Input: part model. Units: mm. Frame: model coordinates. Face numbers are marked on the shaded views. A direction names the side the tool comes from. Give positions to 0.01 mm unless a question says otherwise; leave off trailing zeros. Loops run counter-clockwise (first coordinate to the right, second up) from the corner with the lowest first, then second, coordinate; pieces in that order, holes last. Notation, with made-up numbers: (35, -16) -> (82, -16) arc R15 cw to (82, 5) -> close; hole circle Ø10 at (-22.75, 68.5). An arc over 180 degrees is marked (long way). One line per question, with ' | ' between items.
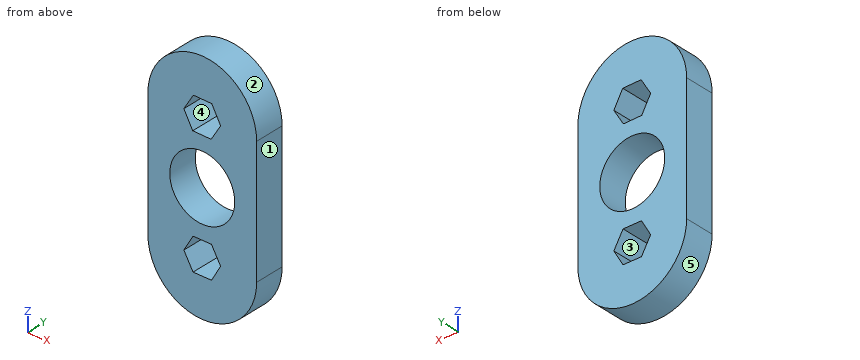
from build123d import *

# Parameters (mm, degrees)
F0_R     = 10.9
F1_DEPTH = 10


with BuildPart() as f1:
    # F0 (on Front) → F1 (new body)
    with BuildSketch(Plane.XZ):
        with BuildLine():
            Line((-18.25, 21), (-18.25, -21))
            ThreePointArc((-18.25, -21), (0, -39.25), (18.25, -21))
            Line((18.25, -21), (18.25, 21))
            ThreePointArc((18.25, 21), (0, 39.25), (-18.25, 21))
        make_face()
        Polygon((-6.177648, -21), (-3.088824, -15.65), (3.088824, -15.65), (6.177648, -21), (3.088824, -26.35), (-3.088824, -26.35), align=None, mode=Mode.SUBTRACT)
        Polygon((-2.979001, 26.411921), (3.19736, 26.285851), (6.176361, 20.87393), (2.979001, 15.588079), (-3.19736, 15.714149), (-6.176361, 21.12607), align=None, mode=Mode.SUBTRACT)
        Circle(F0_R, mode=Mode.SUBTRACT)
    extrude(amount=F1_DEPTH)


solid = f1.part
1. Section query B-B (y = -9). Output: boundary loops of the cut face in (x, z), then the cut area to 3 significant figures.
Determined:
outline: (-18.25, -21) arc R18.25 ccw to (18.25, -21) -> (18.25, 21) arc R18.25 ccw to (-18.25, 21) -> close; hole circle Ø21.8 at (0, 0); hole (-6.18, -21) -> (-3.09, -26.35) -> (3.09, -26.35) -> (6.18, -21) -> (3.09, -15.65) -> (-3.09, -15.65) -> close; hole (-6.18, 21.13) -> (-3.2, 15.71) -> (2.98, 15.59) -> (6.18, 20.87) -> (3.2, 26.29) -> (-2.98, 26.41) -> close | area: 2,010 mm2
2. Section query A-A (z = 0). Output: boundary loops of the cut face in (x, y), then the cut area to 3 significant figures.
Determined:
outline: (-18.25, -10) -> (-10.9, -10) -> (-10.9, 0) -> (-18.25, 0) -> close; (10.9, -10) -> (18.25, -10) -> (18.25, 0) -> (10.9, 0) -> close | area: 147 mm2
3. Ray query, line 1 along Z through (x, y) = (-2, -1.75); line 2 along Z through (x, y) = (2, -8.5); line 3 along X through (y, z) = (-8.75, 20.5). Return the intervals inside material, ascending. Write a range as from..to.
Determined:
line 1: z = -39.14..-26.35, -15.65..-10.71, 10.71..15.69, 26.39..39.14 | line 2: z = -39.14..-26.35, -15.65..-10.71, 10.71..15.61, 26.31..39.14 | line 3: x = -18.25..-5.83, 5.95..18.25
4. Section query D-D (x = 0). Output: boundary loops of the cut face in (y, z), then the cut area to 3 significant figures.
Determined:
outline: (-10, -39.25) -> (0, -39.25) -> (0, -26.35) -> (-10, -26.35) -> close; (-10, -15.65) -> (0, -15.65) -> (0, -10.9) -> (-10, -10.9) -> close; (-10, 10.9) -> (0, 10.9) -> (0, 15.65) -> (-10, 15.65) -> close; (-10, 26.35) -> (0, 26.35) -> (0, 39.25) -> (-10, 39.25) -> close | area: 353 mm2
5. Pin query (flat end, axial travel): P1, Ø1, axis at y = -3.5, z = -31, coming from the -X side; P2, Ø3, axis at x = 0.5, y = -3, coming from the -Z side; P3, Ø2, axis at x = 7.5, y = -3, coming from the +Z side; P4, Ø1, axis at x = 12.5, z = -13, coming from the +Y side. Return the tip coordinate at first contact, or that it passes through.
Determined:
P1: stops at x = -15.58 | P2: stops at z = -39.25 | P3: stops at z = 38.05 | P4: stops at y = 0
6. Section query C-C (x = 9). Output: boundary loops of the cut face in (y, z).
Determined:
outline: (-10, -36.88) -> (0, -36.88) -> (0, -6.15) -> (-10, -6.15) -> close; (-10, 6.15) -> (0, 6.15) -> (0, 36.88) -> (-10, 36.88) -> close
7. Pull-direction query (Z, two-part tool) for the marked faces 1, 2 and 3; classes: pulls with the +Z half, pulls with the -Z half, needs draft (parallel to the pull), parting line crosses it, or undercut.
Determined:
face 1: needs draft | face 2: pulls with the +Z half | face 3: undercut
8. Reachability of the marked faces 4 and 5 from +Z, -Z, +X, -X, +Y, -Y: full face, straight path, thin tool, end or side. Return the list, or none.
Determined:
face 4: +Y, -Y | face 5: -Z, +Y, -Y
